Geometry check sheet. Reference: the model listing, model coordinates, mm. Face numbers are marked on the shaded views. A direction names the side the tool comes from. Coordinates: 2 decimals unless noted, no trailing zeros. Loops run counter-clockwise (first coordinate to the right, second up) from the corner with the lowest first, then second, coordinate; pieces in that order, holes last. Notation, with made-up numbers: (6, 7) - (56, 7) arc R21 ccw to (56, 42) - close; hole circle Ø5 at (61, 50). An arc over 180 degrees is marked (long way). Write item = value, one per line. Start each with the question number.
Autodesk Inventor part; units mm, degrees
ref_plane "YZ Plane" through (0, 0, 0) normal (1, 0, 0) x (0, 1, 0)
ref_plane "XZ Plane" through (0, 0, 0) normal (0, 1, 0) x (-1, 0, 0)
ref_plane "XY Plane" through (0, 0, 0) normal (0, 0, 1) x (1, 0, 0)
sketch "Sketch1" plane through (0, 0, 0) normal (0, 0, 1) x (1, 0, 0)
  circle A0 centre (0, 0) radius 11.5
  line L0 (-18, -21) -> (18, -21)
  line L1 (21, -18) -> (21, 18)
  line L2 (18, 21) -> (-18, 21)
  line L3 (-21, 18) -> (-21, -18)
  line L4 (-21, -21) -> (21, 21) construction
  line L5 (21, -21) -> (-21, 21) construction
  circle A1 centre (-15.5, 15.5) radius 1.875
  circle A2 centre (15.5, 15.5) radius 1.875
  circle A3 centre (15.5, -15.5) radius 1.875
  circle A4 centre (-15.5, -15.5) radius 1.875
  line L6 (-15.5, 15.5) -> (15.5, 15.5) construction
  line L7 (15.5, 15.5) -> (15.5, -15.5) construction
  line L8 (15.5, -15.5) -> (-15.5, -15.5) construction
  line L9 (-15.5, 15.5) -> (-15.5, -15.5) construction
  line L10 (-15.5, 15.5) -> (15.5, -15.5) construction
  line L11 (15.5, 15.5) -> (0, 0) construction
  circle A5 centre (-23, 4) radius 3.95
  circle A6 centre (23, 4) radius 3.95
  circle A7 centre (-23, 4) radius 11
  circle A8 centre (23, 4) radius 11
  line L12 (0, 126.4593) -> (0, -125.5407)
  line L13 (-111.8366, 0) -> (126.1634, 0)
  circle A9 centre (-48.8366, 35.9593) radius 2.0625
  circle A10 centre (-57.8366, 80.4593) radius 2.0625
  circle A11 centre (-66.8366, 35.9593) radius 2.0625
  circle A12 centre (-66.8366, 60.9593) radius 2.0625
  circle A13 centre (-48.8366, 60.9593) radius 2.0625
  circle A14 centre (63.1634, 35.9593) radius 2.0625
  circle A15 centre (72.1634, 80.4593) radius 2.0625
  circle A16 centre (81.1634, 35.9593) radius 2.0625
  circle A17 centre (81.1634, 60.9593) radius 2.0625
  circle A18 centre (63.1634, 60.9593) radius 2.0625
  circle A19 centre (-48.8366, -35.0407) radius 2.0625
  circle A20 centre (-57.8366, -79.5407) radius 2.0625
  circle A21 centre (-66.8366, -35.0407) radius 2.0625
  circle A22 centre (-66.8366, -60.0407) radius 2.0625
  circle A23 centre (-48.8366, -60.0407) radius 2.0625
  circle A24 centre (63.1634, -35.0407) radius 2.0625
  circle A25 centre (63.1634, -60.0407) radius 2.0625
  circle A26 centre (81.1634, -60.0407) radius 2.0625
  circle A27 centre (81.1634, -35.0407) radius 2.0625
  circle A28 centre (72.1634, -79.5407) radius 2.0625
  line L14 (92.1634, -89.5407) -> (92.1634, 90.4593)
  line L15 (92.1634, 90.4593) -> (-77.8366, 90.4593)
  line L16 (-77.8366, 90.4593) -> (-77.8366, -89.5407)
  line L17 (-77.8366, -89.5407) -> (92.1634, -89.5407)
  circle A29 centre (-48.8366, 35.9593) radius 2.0625
  circle A30 centre (-57.8366, 80.4593) radius 2.0625
  circle A31 centre (-66.8366, 35.9593) radius 2.0625
  circle A32 centre (-66.8366, 60.9593) radius 2.0625
  circle A33 centre (-48.8366, 60.9593) radius 2.0625
  circle A34 centre (63.1634, 35.9593) radius 2.0625
  circle A35 centre (72.1634, 80.4593) radius 2.0625
  circle A36 centre (81.1634, 35.9593) radius 2.0625
  circle A37 centre (81.1634, 60.9593) radius 2.0625
  circle A38 centre (63.1634, 60.9593) radius 2.0625
  circle A39 centre (-48.8366, -35.0407) radius 2.0625
  circle A40 centre (-57.8366, -79.5407) radius 2.0625
  circle A41 centre (-66.8366, -35.0407) radius 2.0625
  circle A42 centre (-66.8366, -60.0407) radius 2.0625
  circle A43 centre (-48.8366, -60.0407) radius 2.0625
  circle A44 centre (63.1634, -35.0407) radius 2.0625
  circle A45 centre (63.1634, -60.0407) radius 2.0625
  circle A46 centre (81.1634, -60.0407) radius 2.0625
  circle A47 centre (81.1634, -35.0407) radius 2.0625
  circle A48 centre (72.1634, -79.5407) radius 2.0625
  line L18 (92.1634, -89.5407) -> (92.1634, 90.4593)
  line L19 (92.1634, 90.4593) -> (-77.8366, 90.4593)
  line L20 (-77.8366, 90.4593) -> (-77.8366, -89.5407)
  line L21 (-77.8366, -89.5407) -> (92.1634, -89.5407)
  arc A49 (-18, 21) -> (-21, 18) centre (-18, 18) ccw
  arc A50 (21, 18) -> (18, 21) centre (18, 18) ccw
  arc A51 (18, -21) -> (21, -18) centre (18, -18) ccw
  arc A52 (-21, -18) -> (-18, -21) centre (-18, -18) ccw
  line L22 (-28.0915, -5.7507) -> (-21, -9.4536)
  line L23 (-28.0915, 13.7507) -> (-21, 17.4536)
  line L24 (28.0915, -5.7507) -> (21, -9.4536)
  line L25 (28.0915, 13.7507) -> (21, 17.4536)
  circle A53 centre (-23, 4) radius 5.5
  circle A54 centre (23, 4) radius 5.5
  dimension "d0" = 23
  dimension "d1" = 3.75
  dimension "d2" = 31
  dimension "d3" = 31
  dimension "d4" = 22
  dimension "d5" = 42
  dimension "d6" = 42
  dimension "d7" = 23
  dimension "d8" = 4
  dimension "d9" = 7.9
  dimension "d10" = 3
  dimension "d11" = 8
  dimension "d12" = 11
extrude "Extrusion1" add sketch "Sketch1" along normal blind 4 contours L13 A8 L1 A51 L0 L12 A0 | A0 L12 L2 A50 L1 A8 L13 | A0 L13 A7 L3 A49 L2 L12 | L12 L0 A52 L3 A7 L13 A0 | L13 A54 L1 A8 | A8 L1 A54 L13 | A8 L13 A54 L1 | L1 L25 A8 | A8 L24 L1 | L1 A54 L13 A8 | A54 L1 A6 L13 | L13 L1 A54 | L13 A53 L3 A7 | A7 L3 A53 L13 | A54 L13 L1 A6 | L1 L13 A54 | A7 L13 A53 L3 | L3 L22 A7 | A53 L3 L13 | L13 L3 A5 A53 | A6 L1 | L1 A6 | A53 L13 L3 | A7 L23 L3 | L3 A53 L13 A7 | L13 A53 L3 A5 | A5 L3 | L3 A5
sketch "Sketch2" plane through (0, 0, 4) normal (0, 0, 1) x (1, 0, 0)
  circle A0 centre (0, 0) radius 11.5
  circle A1 centre (-15.5, -15.5) radius 1.875
  circle A2 centre (15.5, -15.5) radius 1.875
  circle A3 centre (15.5, 15.5) radius 1.875
  circle A4 centre (-15.5, 15.5) radius 1.875
  line L0 (28.0915, 13.7507) -> (21, 17.4536)
  line L1 (21, 17.4536) -> (21, 18)
  arc A5 (21, 18) -> (18, 21) centre (18, 18) ccw
  line L2 (18, 21) -> (-18, 21)
  arc A6 (-18, 21) -> (-21, 18) centre (-18, 18) ccw
  line L3 (-21, 18) -> (-21, 17.4536)
  line L4 (-21, 17.4536) -> (-28.0915, 13.7507)
  arc A7 (-28.0915, 13.7507) -> (-28.0915, -5.7507) centre (-23, 4) ccw
  line L5 (-28.0915, -5.7507) -> (-21, -9.4536)
  line L6 (-21, -9.4536) -> (-21, -18)
  arc A8 (-21, -18) -> (-18, -21) centre (-18, -18) ccw
  line L7 (-18, -21) -> (18, -21)
  arc A9 (18, -21) -> (21, -18) centre (18, -18) ccw
  line L8 (21, -18) -> (21, -9.4536)
  line L9 (21, -9.4536) -> (28.0915, -5.7507)
  arc A10 (28.0915, -5.7507) -> (28.0915, 13.7507) centre (23, 4) ccw
  circle A11 centre (23, 4) radius 5.5
  circle A12 centre (-23, 4) radius 5.5
  circle A13 centre (23, 4) radius 3.95
  circle A14 centre (-23, 4) radius 3.95
  dimension "d15" = 11
  dimension "d16" = 7.9
  dimension "d17" = 7.9
  dimension "d18" = 11
extrude "Extrusion2" add sketch "Sketch2" along normal blind 8.75 contours A13 | A14
extrude "Extrusion3" add sketch "Sketch2" along normal blind 1.75 contours A11 | A12
fillet "Fillet1" radius 0.5 2 edges at (19.05, 4, 12.75) (-26.95, 4, 12.75)
sketch "Sketch3" plane through (23, 4, 12.75) normal (0, 0, 1) x (1, 0, 0)
  circle A0 centre (0, 0) radius 3.45
  circle A1 centre (-46, 0) radius 3.45
  circle A2 centre (0, 0) radius 1.925
  circle A3 centre (-46, 0) radius 1.925
  point P0 (-23, -4)
  dimension "d24" = 3.85
extrude "Extrusion4" cut sketch "Sketch3" against normal blind 8 contours A2 | A3
properties part number "Stepper Atachments"
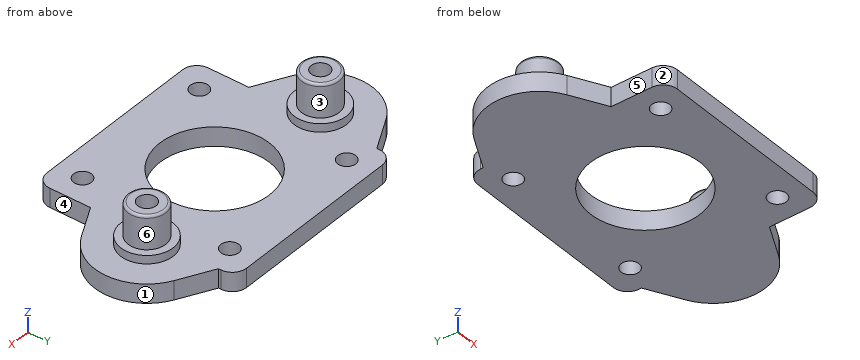
(1) Sectioned sample at A-A on x = 0. Enter the section's corners in (y, z), plus the area to 3 significant figures.
(2) Sectioned sample at B-B on x = -15.5. Enter the section's corners in (y, z) (3 decimals).
(3) Sectioned sample at D-D on y = 15.5. Enter the section's corners in (x, z) (3 decimals).
(4) Scan lines: line 1 (Y direction, x = -15.5, z = 2.5) (3 decimals); line 2 (Y direction, x = 23, z = 9) (3 decimals); line 3 (X direction, y = -15, z = 3.75). Record each from-to range of solid material in increasing order.
(5) Draft check along X on the marked faces 1, 2 and 3. Enter one of: pulls with the +X half, pulls with the -X half, needs draft (parallel to the pull), parting line crosses it, or undercut.
(6) Sectioned sample at C-C on z = 8.25. Enter the section's corners in (x, y) (3 decimals).
(7) Depth check by flat-ended pin: pin 1 (3 mm diameter, centred on y = -12.5, z = 2.5, fed in from +X); pin 2 (4 mm diameter, centred on x = 22, z = 4.5, fed in from -Y); pin 3 (1.5 mm diameter, centred on y = 6.5, z = 5.5, fed in from +X). Enter the tip coordinate at first touch or a pass-through.
(8) Tool access check on the marked faces 4, 5 and 6. Record the directions out of +Z, -Z, +X, -X, +Y, -Y that give a thin tool (end or side, any length) a straight path to the whole face; none if there is none.
Working result:
q1.outline = (-21, 0) - (-11.5, 0) - (-11.5, 4) - (-21, 4) - close; (11.5, 0) - (21, 0) - (21, 4) - (11.5, 4) - close
q1.area = 76.0 mm2
q2.outline = (-21, 0) - (-17.375, 0) - (-17.375, 4) - (-21, 4) - close; (-13.625, 0) - (13.625, 0) - (13.625, 4) - (-13.625, 4) - close; (17.375, 0) - (21, 0) - (21, 4) - (17.375, 4) - close
q3.outline = (-24.741, 0) - (-17.375, 0) - (-17.375, 4) - (-24.741, 4) - close; (-13.625, 0) - (13.625, 0) - (13.625, 4) - (-13.625, 4) - close; (17.375, 0) - (24.741, 0) - (24.741, 4) - (17.375, 4) - close
q4.line_1 = -21 to -17.375, -13.625 to 13.625, 17.375 to 21
q4.line_2 = 0.05 to 2.075, 5.925 to 7.95
q4.line_3 = -21 to -17.31, -13.69 to 13.69, 17.31 to 21
q5.face_1 = pulls with the +X half
q5.face_2 = pulls with the -X half
q5.face_3 = undercut
q6.outline = circle Ø7.9 at (-23, 4); circle Ø7.9 at (23, 4); hole circle Ø3.85 at (-23, 4); hole circle Ø3.85 at (23, 4)
q7.pin_1 = 21
q7.pin_2 = -20.18
q7.pin_3 = 28.21
q8.face_4 = +Z, -Z, +X, -Y
q8.face_5 = +Z, -Z, -X, -Y
q8.face_6 = +Z
